from build123d import *

# Parameters (mm, degrees)
SKETCH1_R           = 1.5
SKETCH1_R_2         = 5.999572562
SKETCH1_R_3         = 6
BOSS_EXTRUDE1_DEPTH = 3.175
FILLET1_R           = 10
FILLET2_R           = 5
FILLET3_R           = 5
FILLET4_R           = 5
FILLET5_R           = 2


with BuildPart() as part:
    # Sketch1 → Boss-Extrude1 (new body)
    with BuildSketch(Plane.XY):
        with BuildLine():
            ThreePointArc((0, 24.142135624), (0.761204675, 20.3153013), (2.928932188, 17.071067812))
            Line((2.928932188, 17.071067812), (17.071067812, 2.928932188))
            ThreePointArc((17.071067812, 2.928932188), (20.3153013, 0.761204675), (24.142135624, 0))
            Line((24.142135624, 0), (420.357864376, 0))
            ThreePointArc((420.357864376, 0), (424.1846987, 0.761204675), (427.428932188, 2.928932188))
            Line((427.428932188, 2.928932188), (441.571067812, 17.071067812))
            ThreePointArc((441.571067812, 17.071067812), (443.738795325, 20.3153013), (444.5, 24.142135624))
            Line((444.5, 24.142135624), (444.5, 72.55))
            ThreePointArc((444.5, 72.55), (441.571067812, 79.621067812), (434.5, 82.55))
            Line((434.5, 82.55), (10, 82.55))
            ThreePointArc((10, 82.55), (2.928932188, 79.621067812), (0, 72.55))
            Line((0, 72.55), (0, 24.142135624))
        make_face()
        with Locations((124.487832174, 7.5)):
            Circle(SKETCH1_R, mode=Mode.SUBTRACT)
        with BuildLine():
            ThreePointArc((12.928932188, 21.213203436), (10.761204675, 24.457436924), (10, 28.284271247))
            Line((10, 28.284271247), (10, 56.550427438))
            Line((10, 56.550427438), (34.800427438, 31.75))
            Line((34.800427438, 31.75), (34.800427438, 10))
            Line((34.800427438, 10), (28.284271247, 10))
            ThreePointArc((28.284271247, 10), (24.457436924, 10.761204675), (21.213203436, 12.928932188))
            Line((21.213203436, 12.928932188), (12.928932188, 21.213203436))
        make_face(mode=Mode.SUBTRACT)
        with Locations((50.8, 31.75)):
            Circle(SKETCH1_R_2, mode=Mode.SUBTRACT)
        with BuildLine():
            Line((199.331464685, 38.668535315), (206.25, 31.75))
            Line((206.25, 31.75), (206.25, 10))
            Line((206.25, 10), (131.558899986, 10))
            ThreePointArc((131.558899986, 10), (124.487832174, 15), (117.416764362, 10))
            Line((117.416764362, 10), (66.799572562, 10))
            Line((66.799572562, 10), (199.331464685, 38.668535315))
        make_face(mode=Mode.SUBTRACT)
        with Locations((320.012167826, 7.5)):
            Circle(SKETCH1_R, mode=Mode.SUBTRACT)
        with BuildLine():
            Line((238.25, 10), (238.25, 31.75))
            Line((238.25, 31.75), (245.168535315, 38.668535315))
            Line((245.168535315, 38.668535315), (377.700427438, 10))
            Line((377.700427438, 10), (327.083235638, 10))
            ThreePointArc((327.083235638, 10), (320.012167826, 15), (312.941100014, 10))
            Line((312.941100014, 10), (238.25, 10))
        make_face(mode=Mode.SUBTRACT)
        with Locations((222.25, 31.75)):
            Circle(SKETCH1_R_3, mode=Mode.SUBTRACT)
        with Locations((393.7, 31.75)):
            Circle(SKETCH1_R_2, mode=Mode.SUBTRACT)
        with BuildLine():
            Line((434.5, 56.550427438), (434.5, 28.284271247))
            ThreePointArc((434.5, 28.284271247), (433.738795325, 24.457436924), (431.571067812, 21.213203436))
            Line((431.571067812, 21.213203436), (423.286796564, 12.928932188))
            ThreePointArc((423.286796564, 12.928932188), (420.042563076, 10.761204675), (416.215728753, 10))
            Line((416.215728753, 10), (409.699572562, 10))
            Line((409.699572562, 10), (409.699572562, 31.75))
            Line((409.699572562, 31.75), (434.5, 56.550427438))
        make_face(mode=Mode.SUBTRACT)
        Polygon((50.8, 47.749572562), (25.999572562, 72.55), (75.600427438, 72.55), align=None, mode=Mode.SUBTRACT)
        Polygon((181.449572562, 56.550427438), (66.799572562, 31.75), (107.599572562, 72.55), (165.45, 72.55), align=None, mode=Mode.SUBTRACT)
        Polygon((247.05, 72.55), (222.25, 47.75), (197.45, 72.55), align=None, mode=Mode.SUBTRACT)
        with Locations((10, 75.05)):
            Circle(SKETCH1_R, mode=Mode.SUBTRACT)
        Polygon((263.050427438, 56.550427438), (279.05, 72.55), (336.900427438, 72.55), (377.700427438, 31.75), align=None, mode=Mode.SUBTRACT)
        Polygon((418.500427438, 72.55), (393.7, 47.749572562), (368.899572562, 72.55), align=None, mode=Mode.SUBTRACT)
        with Locations((434.5, 75.05)):
            Circle(SKETCH1_R, mode=Mode.SUBTRACT)
    extrude(amount=BOSS_EXTRUDE1_DEPTH)

    # Fillet1
    fillet1_edges = [part.edges().sort_by_distance(p)[0] for p in [
        (34.800427438, 31.75, 1.5875),
        (409.699572562, 31.75, 1.5875),
        (336.900427438, 72.55, 1.5875),
        (279.05, 72.55, 1.5875),
        (165.45, 72.55, 1.5875),
        (107.599572562, 72.55, 1.5875),
    ]]
    fillet(fillet1_edges, radius=FILLET1_R)

    # Fillet2
    fillet2_edges = [part.edges().sort_by_distance(p)[0] for p in [
        (245.168535315, 38.668535315, 1.5875),
        (238.25, 31.75, 1.5875),
        (238.25, 10, 1.5875),
        (34.800427438, 10, 1.5875),
        (409.699572562, 10, 1.5875),
        (206.25, 10, 1.5875),
        (206.25, 31.75, 1.5875),
        (199.331464685, 38.668535315, 1.5875),
    ]]
    fillet(fillet2_edges, radius=FILLET2_R)

    # Fillet3
    fillet3_edges = [part.edges().sort_by_distance(p)[0] for p in [
        (222.25, 47.75, 1.5875),
        (247.05, 72.55, 1.5875),
        (197.45, 72.55, 1.5875),
    ]]
    fillet(fillet3_edges, radius=FILLET3_R)

    # Fillet4
    fillet4_edges = [part.edges().sort_by_distance(p)[0] for p in [
        (10, 56.550427438, 1.5875),
        (434.5, 56.550427438, 1.5875),
        (75.600427438, 72.55, 1.5875),
        (25.999572562, 72.55, 1.5875),
        (50.8, 47.749572562, 1.5875),
        (393.7, 47.749572562, 1.5875),
        (418.500427438, 72.55, 1.5875),
        (368.899572562, 72.55, 1.5875),
    ]]
    fillet(fillet4_edges, radius=FILLET4_R)

    # Fillet5
    fillet5_edges = [part.edges().sort_by_distance(p)[0] for p in [
        (377.700427438, 10, 1.5875),
        (377.700427438, 31.75, 1.5875),
        (263.050427438, 56.550427438, 1.5875),
        (66.799572562, 31.75, 1.5875),
        (181.449572562, 56.550427438, 1.5875),
        (66.799572562, 10, 1.5875),
    ]]
    fillet(fillet5_edges, radius=FILLET5_R)


solid = part.part
The model under review builds one solid part; all positions refer to its coordinate system, in mm. A direction names the side the tool comes from. Coordinates: 2 decimals unless noted, no trailing zeros. Put each result on its own line as item: value. Start each with the question number.
Q1. The part is to be moulded in two halves that separate along X. For faces 3 (the cylindrical face through (441.65, 79.54, 1.57)), 4 (the cylindrical face through (3.01, 79.7, 1.57)), 5 (the flat face through (356.13, 53.32, 1.57)), 6 (the flat face through (17.13, 17.01, 1.57)), say which applies: +X half, -X half, draft (parallel to the pull), parting line (faces both ways), or undercut.
Q2. Wall thickness on line 1 (Y direction, x = 223, z = 2.6); line 2 (X direction, y = 70.5, z = 3); line 3 (Y direction, x = 84, z = 2.95): over which ranges is each line inside the solid? List them lowest first.
Q3. For faces 1 (the flat face through (319.577, 44.323, 1.565)), 2 (the flat face through (434.4, 9.9, 1.6)), list the 3-axis set-ups (+Z, -Z, +X, -X, +Y, -Y) from which the entire face can be reached by the end or side of a thin tool; tool diameter is ignored.
Q4. Clearance check with a flat-ended pin moving along its axis: pin 1 (2.5 mm diameter, centred on x = 320.01, y = 7.5, fed in from +Z). State where the tip first meets the part, or that it passes through.
Q5. Add section A-A (z = 0.8). Count the separate pieces of the cut face and the enclosed holes in it, and give its area (3 significant figures).
Answers:
1. face 3: +X half
1. face 4: -X half
1. face 5: undercut
1. face 6: undercut
2. line 1: y = 0 to 25.8, 37.7 to 49.88, 72.55 to 82.55
2. line 2: x = 0 to 34.03, 67.57 to 105.68, 167.37 to 205.48, 239.02 to 277.13, 338.82 to 376.93, 410.47 to 444.5
2. line 3: y = 0 to 10.68, 13.32 to 35.47, 48.95 to 82.55
3. face 1: +Z, -Z
3. face 2: +Z, -Z, +X, -Y
4. pin 1: passes through
5. separate pieces: 1
5. enclosed holes: 16
5. area: 24,300 mm^2
